Here's how the part is built. I have some questions about the finished solid (model axes, mm). A direction names the side the tool comes from. Give positions to 0.01 mm unless a question says otherwise; leave off trailing zeros. Loops run counter-clockwise (first coordinate to the right, second up) from the corner with the lowest first, then second, coordinate; pieces in that order, holes last. Notation, with made-up numbers: (77, 0) - (120, 0) arc R23 ccw to (120, 14) - close; hole circle Ø1 at (74, -18). An arc over 180 degrees is marked (long way). Return JSON: item names as keys, results as strings. Group by question number.
(1) I need wall thicknesses on probe 1 along Z at (x, y) = (-54, 90.5); probe 2 along X at (y, z) = (47, -35.5); probe 3 along Y at (x, z) = (169, 60.5). Which ranges of each line are inside material? Lowest first, please. Write a range as [from, to].
(2) If we mould it in two halves opening along Z, with no side actions, what happens to faces 1 (the cylindrical face through (213.15, 127.99, -1.95)), 2 (the flat face through (-3, 65, 139.5)), 3 (the flat face through (206, 65, 2)), 4 (the flat face through (-3, 65, -139.5))? For each: released by +Z, released by -Z, zero draft, split by the parting line, or undercut.
(3) On a 3-axis mill with a long thin cutter (end or side, diameter ignored), from which of +Z, -Z, +X, -X, +Y, -Y can I reach the whole of each face in a straight line? I mean faces 5 (the flat face through (-3, 65, -129.5)), 6 (the cylindrical face through (-213.15, 127.99, -1.95)). Say none if no direction works.
(4) If we section it at C-C (z = 25): Please give me the cut outline in (x, y), then the cut area to 3 significant figures.
(5) If we section it at A-A (y = 115.5): Please give me the cut outline in (x, z), then the cut area to 3 significant figures.
(6) If we section it at B-B (x = -162.5): Please give me the cut outline in (y, z), then the cut area to 3 significant figures.
```python
from build123d import *

# Parameters (mm, degrees)
ESQUISSE1_W        = 432
ESQUISSE1_H        = 279
BOSS_EXTRU_1_DEPTH = 131
CONG_1_R           = 10
COQUE1_START       = -206
COQUE1_OUTLINE_W   = 111
COQUE1_OUTLINE_H   = 259
COQUE1_DEPTH       = 412


# Read off the part's stored shape, not the designer's step: Coque1
with BuildPart() as part:
    # Esquisse1 → Boss.-Extru.1 (new body)
    with BuildSketch(Plane(origin=(0, 0, 0), x_dir=(1, 0, 0), z_dir=(0, 1, 0))):
        Rectangle(ESQUISSE1_W, ESQUISSE1_H)
    extrude(amount=BOSS_EXTRU_1_DEPTH)

    # Congé1
    cong_1_edges = [part.edges().sort_by_distance(p)[0] for p in [
        (-216, 131, 0),
        (216, 131, 0),
        (-216, 0, 0),
        (216, 0, 0),
    ]]
    fillet(cong_1_edges, radius=CONG_1_R)

    # Coque1 outline → Coque1 (cut)
    with BuildSketch(Plane.YZ.offset(COQUE1_START)):
        with Locations((65.5, 0)):
            Rectangle(COQUE1_OUTLINE_W, COQUE1_OUTLINE_H)
    extrude(amount=COQUE1_DEPTH, mode=Mode.SUBTRACT)


solid = part.part
```
Values:
{
 "1": {"probe 1": "[-139.5, -129.5], [129.5, 139.5]", "probe 2": "[-216, -206], [206, 216]", "probe 3": "[0, 10], [121, 131]"},
 "2": {"face 1": "zero draft", "face 2": "released by +Z", "face 3": "undercut", "face 4": "released by -Z"},
 "3": {"face 5": "none", "face 6": "+Z, -Z, -X, +Y"},
 "4": {"outline": "(-216, 10) arc R10 ccw to (-206, 0) - (206, 0) arc R10 ccw to (216, 10) - (216, 121) arc R10 ccw to (206, 131) - (-206, 131) arc R10 ccw to (-216, 121) - close; hole (-206, 10) - (206, 10) - (206, 121) - (-206, 121) - close", "area": "10,800 mm2"},
 "5": {"outline": "(-216, -139.5) - (216, -139.5) - (216, 139.5) - (-216, 139.5) - close; hole (-206, -129.5) - (206, -129.5) - (206, 129.5) - (-206, 129.5) - close", "area": "13,800 mm2"},
 "6": {"outline": "(0, -139.5) - (131, -139.5) - (131, 139.5) - (0, 139.5) - close; hole (10, -129.5) - (121, -129.5) - (121, 129.5) - (10, 129.5) - close", "area": "7,800 mm2"}
}
